Work out the finished part from the listing and answer in its coordinate system (mm). A direction names the side the tool comes from. Round coordinates to 2 decimals unless told otherwise and drop trailing zeros. Order: outer loops, then holes, each group sorted by start corner. A loop starts at its lowest first (then second) coordinate and runs counter-clockwise, first axis right, second up. Notation, with made-up numbers: (74.5, 67.5) - (80.5, 67.5) arc R13 cw to (80.5, 83.5) - close; hole circle Ø10 at (4, -14.75). An arc over 180 degrees is marked (long way). Use CSV: the item, a comma, the result in double quotes.
from build123d import *

# Parameters (mm, degrees)
SKETCH1_R           = 50
BOSS_EXTRUDE1_DEPTH = 30
SKETCH2_R           = 30
BOSS_EXTRUDE2_DEPTH = 30
SKETCH3_R           = 10
BOSS_EXTRUDE3_DEPTH = 80
SKETCH7_R           = 30
BOSS_EXTRUDE4_DEPTH = 10
SKETCH8_R           = 10
BOSS_EXTRUDE5_DEPTH = 10
SKETCH9_R           = 30
BOSS_EXTRUDE6_DEPTH = 10
SKETCH10_R          = 10
BOSS_EXTRUDE7_DEPTH = 10


with BuildPart() as part:
    # Sketch1 → Boss-Extrude1 (new body)
    with BuildSketch(Plane(origin=(0, 0, 0), x_dir=(0, 0, -1), z_dir=(1, 0, 0))):
        Circle(SKETCH1_R)
    boss_extrude1 = extrude(amount=BOSS_EXTRUDE1_DEPTH)

    # Sketch2 → Boss-Extrude2 (add)
    with BuildSketch(Plane(origin=(30, 0, 0), x_dir=(0, 0, -1), z_dir=(1, 0, 0))):
        Circle(SKETCH2_R)
    boss_extrude2 = extrude(amount=BOSS_EXTRUDE2_DEPTH)

    # Sketch3 → Boss-Extrude3 (add)
    with BuildSketch(Plane(origin=(60, 0, 0), x_dir=(0, 0, -1), z_dir=(1, 0, 0))):
        Circle(SKETCH3_R)
    boss_extrude3 = extrude(amount=BOSS_EXTRUDE3_DEPTH)

    # Mirror1: Boss-Extrude1, Boss-Extrude2, Boss-Extrude3 across plane
    add(boss_extrude1.mirror(Plane(origin=(0, 0, 0), x_dir=(0, 0, 1), z_dir=(1, 0, 0))))
    add(boss_extrude2.mirror(Plane(origin=(0, 0, 0), x_dir=(0, 0, 1), z_dir=(1, 0, 0))))
    add(boss_extrude3.mirror(Plane(origin=(0, 0, 0), x_dir=(0, 0, 1), z_dir=(1, 0, 0))))

    # Sketch7 → Boss-Extrude4 (add)
    with BuildSketch(Plane.ZY.offset(60)):
        Circle(SKETCH7_R)
    extrude(amount=BOSS_EXTRUDE4_DEPTH)

    # Sketch8 → Boss-Extrude5 (add)
    with BuildSketch(Plane.ZY.offset(140)):
        Circle(SKETCH8_R)
    extrude(amount=BOSS_EXTRUDE5_DEPTH)

    # Sketch9 → Boss-Extrude6 (add)
    with BuildSketch(Plane(origin=(60, 0, 0), x_dir=(0, 0, -1), z_dir=(1, 0, 0))):
        Circle(SKETCH9_R)
    extrude(amount=BOSS_EXTRUDE6_DEPTH)

    # Sketch10 → Boss-Extrude7 (add)
    with BuildSketch(Plane(origin=(140, 0, 0), x_dir=(0, 0, -1), z_dir=(1, 0, 0))):
        Circle(SKETCH10_R)
    extrude(amount=BOSS_EXTRUDE7_DEPTH)


solid = part.part
(1) For faces 1 (the flat face through (30, -22, -22)), 2 (the flat face through (-30, -22, -22)), 3 (the flat face through (-150, 0, 0)), determine the directions among +Z, -Z, +X, -X, +Y, -Y from which every point of the face is accessible in a straight line to the end or side of a thin tool.
Findings below:
face 1,"+X"
face 2,"-X"
face 3,"+Z, -Z, -X, +Y, -Y"
(2) Find the intervals of material crossed by L1, parallel to X at y = 21, z = 25.5; L2, parallel to Z at x = 18, y = -0.5; L3, parallel to Z at x = -127.5, y = 0, in increasing order. Write a range as from..to.
Findings below:
L1,"x = -30..30"
L2,"z = -50..50"
L3,"z = -10..10"
(3) Find section C-C (x = -130.5). Determine the outline of the cut face in (y, z).
Findings below:
outline,"circle Ø20 at (0, 0)"
(4) Find section A-A (y = 0). Determine the outline of the cut face in (x, z), and give its area (3 significant figures).
Findings below:
outline,"(-150, -10) - (-70, -10) - (-70, -30) - (-30, -30) - (-30, -50) - (30, -50) - (30, -30) - (70, -30) - (70, -10) - (150, -10) - (150, 10) - (70, 10) - (70, 30) - (30, 30) - (30, 50) - (-30, 50) - (-30, 30) - (-70, 30) - (-70, 10) - (-150, 10) - close"
area,"14,000 mm²"
(5) Each of these flat-tipped pins is pushed along its axis until it touches: pin 1 (5 mm diameter, centred on x = 18.5, z = -33, fed in from -Y); pin 2 (8 mm diameter, centred on x = 69.5, y = 15, fed in from +Z); pin 3 (1.5 mm diameter, centred on x = 60, z = -31.5, fed in from -Y); pin 4 (1 mm diameter, centred on x = -59.5, z = 24, fed in from -Y). Where does it stop, or does it pass through?
Findings below:
pin 1,"stops at y = -39.62"
pin 2,"stops at z = 27.91"
pin 3,"passes through"
pin 4,"stops at y = -18.65"
(6) Find section D-D (y = 22). Determine the outline of the cut face in (x, z).
Findings below:
outline,"(-70, -20.4) - (-30, -20.4) - (-30, -44.9) - (30, -44.9) - (30, -20.4) - (70, -20.4) - (70, 20.4) - (30, 20.4) - (30, 44.9) - (-30, 44.9) - (-30, 20.4) - (-70, 20.4) - close"
